```python
from build123d import *

# Parameters (mm, degrees)
CROQUIS2_R              = 12.5
SALIENTE_EXTRUIR1_DEPTH = 50
REDONDEO1_R             = 2
CROQUIS4_R              = 1.5
SALIENTE_EXTRUIR2_DEPTH = 7
CROQUIS5_W              = 0.93235804
CROQUIS5_H              = 2.963644212
SALIENTE_EXTRUIR3_DEPTH = 4
REDONDEO2_R             = 2
CROQUIS6_R              = 0.814443909
CORTAR_EXTRUIR3_DEPTH   = 18


with BuildPart() as part:
    # Croquis2 → Saliente-Extruir1 (new body)
    with BuildSketch(Plane(origin=(0, 0, 0), x_dir=(1, 0, 0), z_dir=(0, 1, 0))):
        with Locations(Location((0, 0, 0), (0, 0, 270))):
            Circle(CROQUIS2_R)
    extrude(amount=SALIENTE_EXTRUIR1_DEPTH)

    # Redondeo1
    redondeo1_edges = [part.edges().sort_by_distance(p)[0] for p in [
        (0, 0, -12.5),
        (0, 50, -12.5),
    ]]
    fillet(redondeo1_edges, radius=REDONDEO1_R)

    # Croquis4 → Saliente-Extruir2 (add)
    with BuildSketch(Plane(origin=(0, 50, 0), x_dir=(1, 0, 0), z_dir=(0, 1, 0))):
        with Locations(Location((0, 0, 0), (0, 0, 270))):
            Circle(CROQUIS4_R)
    extrude(amount=SALIENTE_EXTRUIR2_DEPTH)

    # Croquis5 → Saliente-Extruir3 (add)
    with BuildSketch(Plane(origin=(0, 0, 0), x_dir=(-1, 0, 0), z_dir=(0, -1, 0))):
        with Locations((-5.00245948, 0)):
            Rectangle(CROQUIS5_W, CROQUIS5_H)
        with Locations((5.00245948, 0)):
            Rectangle(CROQUIS5_W, CROQUIS5_H)
    extrude(amount=SALIENTE_EXTRUIR3_DEPTH)

    # Redondeo2
    # the kernel refuses this fillet: 2 mm, written as the material it takes off along each edge
    with BuildSketch(Plane(origin=(-0.46371954, -4, -1.481822106), x_dir=(0, 1, 0), z_dir=(1, 0, 0)), Plane(origin=(10.4686385, -4, 1.481822106), x_dir=(0, 1, 0), z_dir=(-1, 0, 0))) as redondeo2_piece_1:
        with BuildLine():
            CenterArc((REDONDEO2_R, REDONDEO2_R), REDONDEO2_R, 180, 90)
            Line((0, REDONDEO2_R), (0, 0))
            Line((0, 0), (REDONDEO2_R, 0))
        make_face()
    extrude(amount=10.932358039, mode=Mode.SUBTRACT)
    with BuildSketch(Plane(origin=(-10.4686385, -4, 1.481822106), x_dir=(0, 1, 0), z_dir=(1, 0, 0)), Plane(origin=(0.46371954, -4, -1.481822106), x_dir=(0, 1, 0), z_dir=(-1, 0, 0))) as redondeo2_piece_2:
        with BuildLine():
            CenterArc((REDONDEO2_R, -REDONDEO2_R), REDONDEO2_R, 90, 90)
            Line((0, -REDONDEO2_R), (0, 0))
            Line((0, 0), (REDONDEO2_R, 0))
        make_face()
    extrude(amount=10.932358039, mode=Mode.SUBTRACT)

    # Croquis6 → Cortar-Extruir3 (cut)
    with BuildSketch(Plane(origin=(5.4686385, 0, 0), x_dir=(0, 0, -1), z_dir=(1, 0, 0))):
        with Locations((0, -2)):
            Circle(CROQUIS6_R)
    extrude(amount=-CORTAR_EXTRUIR3_DEPTH, mode=Mode.SUBTRACT)


solid = part.part
```
Input: part model. Units: mm. Frame: model coordinates. A direction names the side the tool comes from. Give positions to 0.01 mm unless a question says otherwise; leave off trailing zeros. Order: outer loops, then holes, each group sorted by start corner. A loop starts at its lowest first (then second) coordinate and runs counter-clockwise, first axis right, second up. Notation, with made-up numbers: (78, 1.5) -> (116, 1.5) arc R15 cw to (116, 30.5) -> close; hole circle Ø9 at (82, -29.75). An arc over 180 degrees is marked (long way). Write each question's results on one line, items separated by ' | '. Start each with the question number.
Item 1: Cut plane A-A on x = 0. Return the cut outline in (y, z), then the cut area to 3 significant figures.
Item 2: Line query: line 1 (X direction, y = 10.5, z = 0.25); line 2 (Y direction, x = 5.5, z = 6.25); line 3 (Z direction, x = 10.75, y = 9). Output: solid intervals per line, ascending.
Item 3: Cut plane B-B on y = 41. Return the cut outline in (x, z), then the cut area to 3 significant figures.
Item 4: Contact query for flat-ended pins moving along their axis: P1, Ø1, axis at y = 20, z = 2.5, coming from the +X side; P2, Ø0.9, axis at y = -3, z = 0.5, coming from the +X side; P3, Ø0.7, axis at x = 5, y = -1, coming from the -Z side; P4, Ø1.3, axis at y = -2, z = 0, coming from the +X side. Output: stop coordinate, or through.
Item 5: Mould query, pull axis Y, two halves, no side actions, for faces 6 (the cylindrical face through (-4.996, -1.192, 0.106)), 7 (the cylindrical face through (0.45, 53.45, 1.43)), 8 (the flat face through (0, 0, 0)). Classes: pulls with the +Y half, pulls with the -Y half, needs draft (parallel to the pull), parting line crosses it, or undercut.
Item 6: Set-up query: faces 1 (the cylindrical face through (-5.01, -3.2, 1.08)), 2 (the flat face through (-4.536, -1, 0)), 3 (the cylindrical face through (5, -3.23, -1.06)), 4 (the flat face through (-5.469, -1, 0)), 5 (the flat face through (5.469, -1, 0)). Return all of +Z, -Z, +X, -X, +Y, -Y with unobstructed straight access to the full face (end or side cutting, diameter ignored); none if empty.
Established:
1) outline: (0, -10.5) arc R2 ccw to (2, -12.5) -> (48, -12.5) arc R2 ccw to (50, -10.5) -> (50, -1.5) -> (57, -1.5) -> (57, 1.5) -> (50, 1.5) -> (50, 10.5) arc R2 ccw to (48, 12.5) -> (2, 12.5) arc R2 ccw to (0, 10.5) -> close | area: 1,270 mm^2
2) line 1: -12.5 to 12.5 | line 2: 0 to 50 | line 3: -6.38 to 6.38
3) outline: circle Ø25 at (0, 0) | area: 491 mm^2
4) P1: x = 12.34 | P2: x = 5.47 | P3: z = -1.48 | P4: through
5) face 6: undercut | face 7: needs draft | face 8: pulls with the -Y half
6) face 1: +Z, +X, -X, -Y | face 2: +Z, -Z, -Y | face 3: -Z, +X, -X, -Y | face 4: +Z, -Z, -X, -Y | face 5: +Z, -Z, +X, -Y
